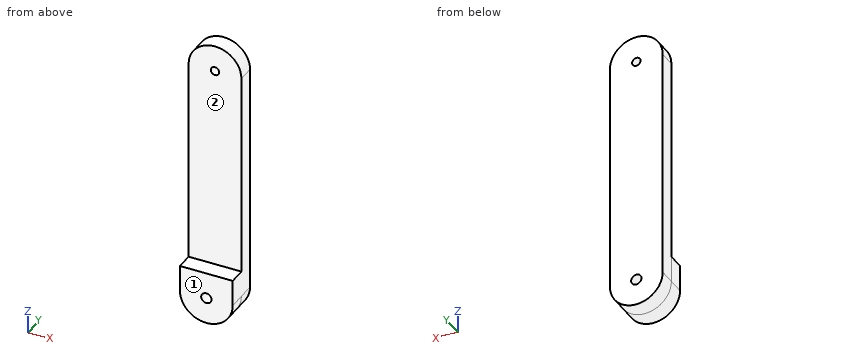
```python
from build123d import *

# Parameters (mm, degrees)
SKETCH1_R               = 12.5
SKETCH1_R_2             = 2.45
BOSS_EXTRUDE1_DEPTH     = 8
CUT_EXTRUDE1_DEPTH      = 124.39570495
CUT_EXTRUDE1_DEPTH_BACK = 124.39570495
SKETCH2_R               = 2
BOSS_EXTRUDE2_START     = 8
BOSS_EXTRUDE2_DEPTH     = 8
CUT_EXTRUDE2_DEPTH      = 125.171252712
CUT_EXTRUDE2_DEPTH_BACK = 125.171252712
SKETCH4_R               = 2.45


with BuildPart() as part:
    # Sketch1 → Boss-Extrude1 (new body)
    # profile 1 of 3: a face of its own
    with BuildSketch(Plane(origin=(0, 0, 0), x_dir=(1, 0, 0), z_dir=(0, 1, 0))):
        with BuildLine():
            Line((12.5, 0), (12.5, 110))
            ThreePointArc((12.5, 110), (0, 97.5), (-12.5, 110))
            Line((-12.5, 110), (-12.5, 0))
            ThreePointArc((-12.5, 0), (0, 12.5), (12.5, 0))
        make_face()
    # profile 2 of 3: a face of its own
    with BuildSketch(Plane(origin=(0, 0, 0), x_dir=(1, 0, 0), z_dir=(0, 1, 0))):
        with Locations((0, 110)):
            Circle(SKETCH1_R)
        with Locations(Location((0, 110, 0), (0, 0, 270))):
            Circle(SKETCH1_R_2, mode=Mode.SUBTRACT)
    # profile 3 of 3: a face of its own
    with BuildSketch(Plane(origin=(0, 0, 0), x_dir=(1, 0, 0), z_dir=(0, 1, 0))):
        Circle(SKETCH1_R)
    extrude(amount=BOSS_EXTRUDE1_DEPTH)

    # Sketch2 → Cut-Extrude1 (cut, two sides: drawn at the far end of the back side and taken through both)
    with BuildSketch(Plane(origin=(0, 8, 0), x_dir=(1, 0, 0), z_dir=(0, 1, 0)).offset(-CUT_EXTRUDE1_DEPTH_BACK)):
        with Locations(Location((0, 0, 0), (0, 0, 270))):
            Circle(SKETCH2_R)
    extrude(amount=CUT_EXTRUDE1_DEPTH + CUT_EXTRUDE1_DEPTH_BACK, mode=Mode.SUBTRACT)

    # Sketch3 → Boss-Extrude2 (add)
    with BuildSketch(Plane.XZ.offset(BOSS_EXTRUDE2_START)):
        with BuildLine():
            Line((12.5, -110), (12.5, -97.5))
            Line((12.5, -97.5), (-12.5, -97.5))
            Line((-12.5, -97.5), (-12.5, -110))
            ThreePointArc((-12.5, -110), (0, -122.5), (12.5, -110))
        make_face()
    extrude(amount=-BOSS_EXTRUDE2_DEPTH)

    # Sketch4 → Cut-Extrude2 (cut, two sides: drawn at the far end of the back side and taken through both)
    with BuildSketch(Plane(origin=(0, 8, 0), x_dir=(1, 0, 0), z_dir=(0, 1, 0)).offset(-CUT_EXTRUDE2_DEPTH_BACK)):
        with Locations(Location((0, 110, 0), (0, 0, 270))):
            Circle(SKETCH4_R)
    extrude(amount=CUT_EXTRUDE2_DEPTH + CUT_EXTRUDE2_DEPTH_BACK, mode=Mode.SUBTRACT)


solid = part.part
```
For this review, take the finished solid that the model builds, in its own axes (mm). Face numbers are marked on the shaded views. A direction names the side the tool comes from. Round coordinates to 2 decimals unless told otherwise and drop trailing zeros. Loops run counter-clockwise (first coordinate to the right, second up) from the corner with the lowest first, then second, coordinate; pieces in that order, holes last.
(1) Clearance check with flat-ended pins moving along their axes: P1, Ø6.5, axis at x = 0, z = 0, coming from the -Y side; P2, Ø4, axis at x = 2, y = -4.5, coming from the +Z side; P3, Ø1.5, axis at x = -7, y = -1.5, coming from the -Z side. State where each tip first meets the part, or that it passes through.
Returned:
P1: stops at y = 0
P2: stops at z = -97.5
P3: stops at z = -120.83
(2) Tool access review of the marked faces 1 and 2: name each direction out of +Z, -Z, +X, -X, +Y, -Y from which nothing blocks a thin tool from reaching the whole face with its end or side.
Returned:
face 1: +Z, -Z, +X, -X, -Y
face 2: +Z, +X, -X, -Y
(3) We need section D-D (x = -10). Give the boundary of the cut face in (y, z), plus the area to 3 significant figures.
Returned:
outline: (-8, -117.5) - (8, -117.5) - (8, 7.5) - (0, 7.5) - (0, -97.5) - (-8, -97.5) - close
area: 1,160 mm2
(4) Wall thickness on line 1 along X through (y, z) = (3, 0); line 2 along Z through (x, y) = (0, -3); line 3 along X through (y, z) = (-2.25, -110): over which ranges is each line inside the solid? List them lowest first.
Returned:
line 1: x = -12.5 to -2, 2 to 12.5
line 2: z = -122.5 to -112.45, -107.55 to -97.5
line 3: x = -12.5 to -2.45, 2.45 to 12.5
(5) We need section B-B (y = -3.5). Give the boundary of the cut face in (x, z).
Returned:
outline: (-12.5, -110) arc R12.5 ccw to (12.5, -110) - (12.5, -97.5) - (-12.5, -97.5) - close; hole circle Ø4.9 at (0, -110)
(6) We need section A-A (x = 0). Give the boundary of the cut face in (y, z).
Returned:
outline: (-8, -122.5) - (8, -122.5) - (8, -112.45) - (-8, -112.45) - close; (-8, -107.55) - (8, -107.55) - (8, -2) - (0, -2) - (0, -97.5) - (-8, -97.5) - close; (0, 2) - (8, 2) - (8, 12.5) - (0, 12.5) - close
(7) We need section C-C (y = 1.5). Give the boundary of the cut face in (x, z), plus the area to 3 significant figures.
Returned:
outline: (-12.5, -110) arc R12.5 ccw to (12.5, -110) - (12.5, 0) arc R12.5 ccw to (-12.5, 0) - close; hole circle Ø4.9 at (0, -110); hole circle Ø4 at (0, 0)
area: 3,210 mm2
